Design review of the part built by this model. Coordinates are the model's own, in mm. Face numbers are marked on the shaded views. Coordinates: 2 decimals unless noted, no trailing zeros. Order: outer loops, then holes, each group sorted by start corner. A loop starts at its lowest first (then second) coordinate and runs counter-clockwise, first axis right, second up. Notation, with made-up numbers: M 54,-15 L 86,-15 A29 cw 86,13 Z; hole C 36.25,5 d10. An arc over 180 degrees is marked long. Answer as a JSON object with one key per item and string values.
from build123d import *

# Parameters (mm, degrees)
BOX_EXTRUDE_DEPTH             = 90
BOX_EXTRUDE_DEPTH_BACK        = 5
SKETCH2_W                     = 140
SKETCH2_H                     = 120
BOX_INNER_CUT_START           = -20
SKETCH3_W                     = 120
SKETCH3_H                     = 100
BOX_INNER_CUT_DEPTH           = 50
SHAFT_CUT_START               = -70
SKETCH6_R                     = 6
SHAFT_CUT_DEPTH               = 20
BEARING_CUTS_INSIDE_BOX_START = -70
SKETCH9_R                     = 8
SKETCH9_R_2                   = 16
BEARING_CUTS_INSIDE_BOX_DEPTH = 10
SCISSOR_CUT_START             = -10
SKETCH11_W                    = 120
SKETCH11_H                    = 14
SCISSOR_CUT_DEPTH             = 156.529453572
LEFT_BEARING_LID_CUT_START    = -10
SKETCH18_R                    = 8
LEFT_BEARING_LID_CUT_DEPTH    = 10
RIGHT_BEARING_LID_CUT_REACH   = 134.382
SKETCH12_R                    = 15
OUTER_EDGES_FILLET_R          = 4


with BuildPart() as part:
    # Sketch2 → BOX_EXTRUDE (new, two sides: drawn at the far end of the back side and taken through both)
    with BuildSketch(Plane(origin=(0, 0, 0), x_dir=(1, 0, 0), z_dir=(0, 1, 0)).offset(-BOX_EXTRUDE_DEPTH_BACK)):
        Rectangle(SKETCH2_W, SKETCH2_H)
    extrude(amount=BOX_EXTRUDE_DEPTH + BOX_EXTRUDE_DEPTH_BACK)

    # Sketch3 → BOX_INNER_CUT (cut)
    with BuildSketch(Plane(origin=(0, 90, 0), x_dir=(1, 0, 0), z_dir=(0, 1, 0)).offset(BOX_INNER_CUT_START)):
        Rectangle(SKETCH3_W, SKETCH3_H)
    extrude(amount=-BOX_INNER_CUT_DEPTH, mode=Mode.SUBTRACT)

    # Sketch6 → SHAFT_CUT (cut)
    with BuildSketch(Plane(origin=(0, 90, 0), x_dir=(1, 0, 0), z_dir=(0, 1, 0)).offset(SHAFT_CUT_START)):
        with Locations(Location((15, 0, 0), (0, 0, 270))):
            Circle(SKETCH6_R)
        with Locations(Location((-15, 0, 0), (0, 0, 90))):
            Circle(SKETCH6_R)
    extrude(amount=-SHAFT_CUT_DEPTH, mode=Mode.SUBTRACT)

    # Sketch9 → BEARING_CUTS_INSIDE_BOX (cut)
    with BuildSketch(Plane(origin=(0, 90, 0), x_dir=(1, 0, 0), z_dir=(0, 1, 0)).offset(BEARING_CUTS_INSIDE_BOX_START)):
        with Locations(Location((15, 0, 0), (0, 0, 270))):
            Circle(SKETCH9_R)
        with Locations(Location((-15, 0, 0), (0, 0, 270))):
            Circle(SKETCH9_R_2)
    extrude(amount=-BEARING_CUTS_INSIDE_BOX_DEPTH, mode=Mode.SUBTRACT)

    # Sketch11 → SCISSOR_CUT (cut, through all)
    with BuildSketch(Plane.XY.offset(60).offset(SCISSOR_CUT_START)):
        with Locations((0, 35)):
            Rectangle(SKETCH11_W, SKETCH11_H)
    extrude(amount=-SCISSOR_CUT_DEPTH, mode=Mode.SUBTRACT)

    # Sketch18 → LEFT_BEARING_LID_CUT (cut)
    with BuildSketch(Plane(origin=(0, 90, 0), x_dir=(1, 0, 0), z_dir=(0, 1, 0)).offset(LEFT_BEARING_LID_CUT_START)):
        with Locations(Location((-15, 0, 0), (0, 0, 270))):
            Circle(SKETCH18_R)
    extrude(amount=-LEFT_BEARING_LID_CUT_DEPTH, mode=Mode.SUBTRACT)

    # Sketch12 → RIGHT_BEARING_LID_CUT (cut, up to next)
    with BuildSketch(Plane(origin=(0, 90, 0), x_dir=(1, 0, 0), z_dir=(0, 1, 0)), mode=Mode.PRIVATE) as right_bearing_lid_cut_sk1:
        with Locations(Location((15, 0, 0), (0, 0, 270))):
            Circle(SKETCH12_R)
    right_bearing_lid_cut_tool1 = extrude(right_bearing_lid_cut_sk1.sketch, amount=-RIGHT_BEARING_LID_CUT_REACH, mode=Mode.PRIVATE) & part.part
    add(right_bearing_lid_cut_tool1.solids().sort_by_distance((15, 90, 0))[0], mode=Mode.SUBTRACT)

    # OUTER_EDGES_FILLET
    outer_edges_fillet_edges = [part.edges().sort_by_distance(p)[0] for p in [
        (-70, 42.5, -60),
        (70, 42.5, -60),
        (70, 42.5, 60),
        (-70, 42.5, 60),
    ]]
    fillet(outer_edges_fillet_edges, radius=OUTER_EDGES_FILLET_R)


solid = part.part
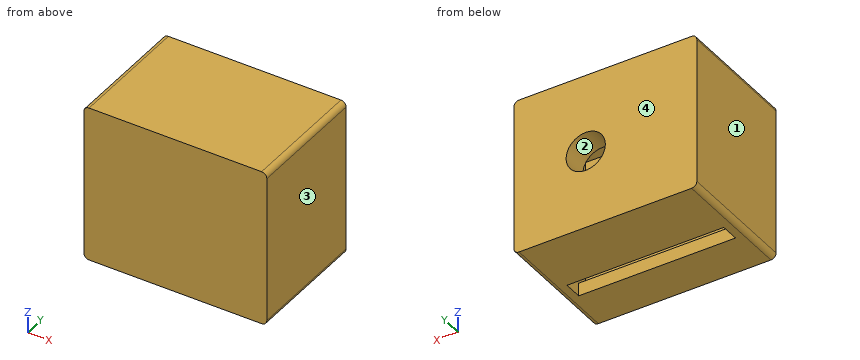
1) Add section A-A (x = 3). State the section outline as (y, z) points.
Taken from the geometry:
{"outline": "M -5,-60 L 28,-60 L 28,-50 L 20,-50 L 20,50 L 70,50 L 70,9 L 90,9 L 90,60 L -5,60 Z; M 42,-60 L 90,-60 L 90,-9 L 70,-9 L 70,-50 L 42,-50 Z"}
2) Add section D-D (x = -43). State the section outline as (y, z) points, and give its area (3 significant figures).
Taken from the geometry:
{"outline": "M -5,-60 L 28,-60 L 28,-50 L 20,-50 L 20,50 L 70,50 L 70,-50 L 42,-50 L 42,-60 L 90,-60 L 90,60 L -5,60 Z", "area": "6,260 mm2"}
3) To check wall thickness, follow L1, parallel to X at y = 17, z = 0; L2, parallel to X at y = 72, z = 0; L3, parallel to Y at x = -51.5, z = -25.5. State the ranges of each line that lie inside material, in increasing order.
Taken from the geometry:
{"L1": "x = -70 to -31, 1 to 7, 23 to 70", "L2": "x = -70 to -23, -7 to 0, 30 to 70", "L3": "y = -5 to 20, 70 to 90"}
4) Add section C-C (y = 16). State the section outline as (x, z) points, and give its area (3 significant figures).
Taken from the geometry:
{"outline": "M -70,-56 A4 ccw -66,-60 L 66,-60 A4 ccw 70,-56 L 70,56 A4 ccw 66,60 L -66,60 A4 ccw -70,56 Z; hole C -15,0 d32; hole C 15,0 d16", "area": "15,800 mm2"}
5) Insertion check: pin 1 Ø6 at (x, z) = (15, -2) entering from +Y; pin 2 Ø18 at (x, z) = (15, 0) entering from +Y. Each pin has a flat end and moves straight along its axis. Give the tip position at first contact, or say it passes through.
Taken from the geometry:
{"pin 1": "stops at y = 0", "pin 2": "stops at y = 20"}
6) Mouldability with a two-part tool opening along X and no side actions: class the marked faces 1, 2, 3 and 4 as released by +X, released by -X, zero draft, split by the parting line, or undercut.
Taken from the geometry:
{"face 1": "released by -X", "face 2": "undercut", "face 3": "released by +X", "face 4": "zero draft"}
7) Add section B-B (z = -18). State the section outline as (x, y) points, and give its area (3 significant figures).
Taken from the geometry:
{"outline": "M -70,-5 L 70,-5 L 70,90 L -70,90 Z; hole M -60,20 L 60,20 L 60,70 L -60,70 Z", "area": "7,300 mm2"}
